The listing builds one solid part. Answer for the finished solid, in the listing's coordinates (mm). Face numbers are marked on the shaded views. A direction names the side the tool comes from. Give positions to 0.01 mm unless a question says otherwise; leave off trailing zeros. Loops run counter-clockwise (first coordinate to the right, second up) from the corner with the lowest first, then second, coordinate; pieces in that order, holes last. Notation, with made-up numbers: (54.25, 66.5) - (105.25, 66.5) arc R24 cw to (105.25, 97.5) - close; hole circle Ø1 at (51, -22). An arc over 180 degrees is marked (long way). One line per item, written item: value. Start each with the question number.
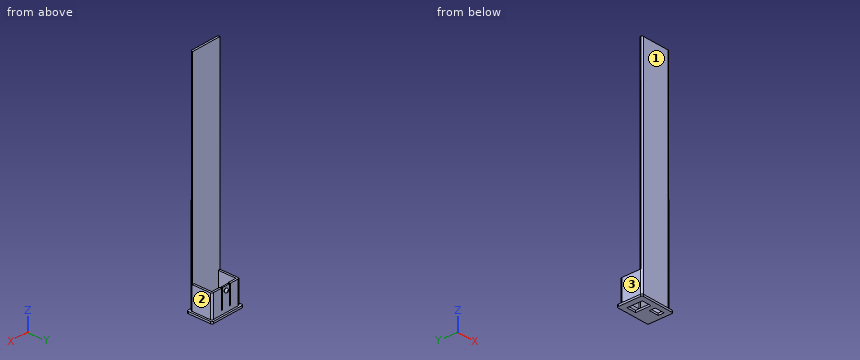
from build123d import *

# Parameters (mm, degrees)
SKETCH1_W           = 25.4
SKETCH1_H           = 17.78
BOSS_EXTRUDE1_DEPTH = 19.05
SKETCH2_W           = 25.4
SKETCH2_H           = 0.79375
BOSS_EXTRUDE2_DEPTH = 165.1
SKETCH3_W           = 28.575
SKETCH3_H           = 20.955
BOSS_EXTRUDE3_DEPTH = 1.5875
SKETCH4_W           = 22.167429019
SKETCH4_H           = 15.39875
CUT_EXTRUDE1_DEPTH  = 19.05
CUT_EXTRUDE2_DEPTH  = 1.5875
SKETCH8_W           = 7.9375
SKETCH8_H           = 4.7625
CUT_EXTRUDE3_DEPTH  = 1.5875
FILLET9_R           = 1.27
FILLET10_R          = 1.27
FILLET11_R          = 1.27
FILLET12_R          = 1.27
FILLET13_R          = 1.27
FILLET14_R          = 1.27
FILLET15_R          = 1.27
FILLET16_R          = 1.27
SKETCH9_W           = 0.79375
SKETCH9_H           = 15.875
CUT_EXTRUDE5_DEPTH  = 1.5875
SKETCH11_W          = 0.79375
SKETCH11_H          = 15.875
CUT_EXTRUDE6_DEPTH  = 1.5875
SKETCH12_W          = 6.50875
SKETCH12_H          = 0.467297544
CUT_EXTRUDE7_DEPTH  = 15.875
SKETCH13_R          = 1.5875
BOSS_EXTRUDE5_DEPTH = 1.5875
FILLET22_R          = 1.27
SKETCH17_W          = 22.167429019
SKETCH17_H          = 19.05
BOSS_EXTRUDE6_DEPTH = 0.79375
SKETCH18_W          = 25.21464302
SKETCH18_H          = 165.1
BOSS_EXTRUDE7_DEPTH = 0.79375


with BuildPart() as part:
    # Sketch1 → Boss-Extrude1 (new body)
    with BuildSketch(Plane.XY):
        with Locations((12.7, 8.89)):
            Rectangle(SKETCH1_W, SKETCH1_H)
    extrude(amount=BOSS_EXTRUDE1_DEPTH)

    # Sketch2 → Boss-Extrude2 (add)
    with BuildSketch(Plane.XY.offset(19.05)):
        with Locations((12.7, 0.396875)):
            Rectangle(SKETCH2_W, SKETCH2_H)
    extrude(amount=BOSS_EXTRUDE2_DEPTH)

    # Sketch3 → Boss-Extrude3 (add)
    with BuildSketch(Plane(origin=(0, 0, 0), x_dir=(-1, 0, 0), z_dir=(0, 0, -1))):
        with Locations((-12.7, 8.89)):
            Rectangle(SKETCH3_W, SKETCH3_H)
    extrude(amount=BOSS_EXTRUDE3_DEPTH)

    # Sketch4 → Cut-Extrude1 (cut)
    with BuildSketch(Plane.XY.offset(19.05)):
        with Locations((12.67121451, 8.493125)):
            Rectangle(SKETCH4_W, SKETCH4_H)
    extrude(amount=-CUT_EXTRUDE1_DEPTH, mode=Mode.SUBTRACT)

    # Sketch5 → Cut-Extrude2 (cut)
    with BuildSketch(Plane(origin=(0, 0, -1.5875), x_dir=(-1, 0, 0), z_dir=(0, 0, -1))):
        Polygon((-11.1125, 15.24), (-11.1125, 8.89), (-11.1125, 2.54), (-3.175, 2.54), (-3.175, 15.24), align=None)
    extrude(amount=-CUT_EXTRUDE2_DEPTH, mode=Mode.SUBTRACT)

    # Sketch8 → Cut-Extrude3 (cut)
    with BuildSketch(Plane(origin=(0, 0, -1.5875), x_dir=(-1, 0, 0), z_dir=(0, 0, -1))):
        with Locations((-19.021212582, 4.92125)):
            Rectangle(SKETCH8_W, SKETCH8_H)
    extrude(amount=-CUT_EXTRUDE3_DEPTH, mode=Mode.SUBTRACT)

    # Fillet9
    fillet9_edges = [part.edges().sort_by_distance(p)[0] for p in [
        (25.4, 17.78, 9.525),
    ]]
    fillet(fillet9_edges, radius=FILLET9_R)

    # Fillet10
    fillet10_edges = [part.edges().sort_by_distance(p)[0] for p in [
        (0, 17.78, 9.525),
    ]]
    fillet(fillet10_edges, radius=FILLET10_R)

    # Fillet11
    # the kernel refuses this fillet: 1.27 mm, written as the material it takes off along each edge
    with BuildSketch(Plane(origin=(25.4, 0, 0), x_dir=(0, 1, 0), z_dir=(0, 0, 1))) as fillet11_piece_1:
        with BuildLine():
            CenterArc((FILLET11_R, FILLET11_R), FILLET11_R, 180, 90)
            Line((0, FILLET11_R), (0, 0))
            Line((0, 0), (FILLET11_R, 0))
        make_face()
    extrude(amount=187.325, mode=Mode.SUBTRACT)

    # Fillet12
    # the kernel refuses this fillet: 1.27 mm, written as the material it takes off along each edge
    with BuildSketch(Plane(origin=(0, 0, 187.325), x_dir=(0, 1, 0), z_dir=(0, 0, -1))) as fillet12_piece_1:
        with BuildLine():
            CenterArc((FILLET12_R, FILLET12_R), FILLET12_R, 180, 90)
            Line((0, FILLET12_R), (0, 0))
            Line((0, 0), (FILLET12_R, 0))
        make_face()
    extrude(amount=187.325, mode=Mode.SUBTRACT)

    # Fillet13
    fillet13_edges = [part.edges().sort_by_distance(p)[0] for p in [
        (-1.5875, -1.5875, -0.79375),
    ]]
    fillet(fillet13_edges, radius=FILLET13_R)

    # Fillet14
    fillet14_edges = [part.edges().sort_by_distance(p)[0] for p in [
        (-1.5875, 19.3675, -0.79375),
    ]]
    fillet(fillet14_edges, radius=FILLET14_R)

    # Fillet15
    fillet15_edges = [part.edges().sort_by_distance(p)[0] for p in [
        (26.9875, -1.5875, -0.79375),
    ]]
    fillet(fillet15_edges, radius=FILLET15_R)

    # Fillet16
    fillet16_edges = [part.edges().sort_by_distance(p)[0] for p in [
        (26.9875, 19.3675, -0.79375),
    ]]
    fillet(fillet16_edges, radius=FILLET16_R)

    # Sketch9 → Cut-Extrude5 (cut)
    with BuildSketch(Plane(origin=(0, 17.78, 0), x_dir=(1, 0, 0), z_dir=(0, 1, 0))):
        with Locations((16.271875, -11.1125)):
            Rectangle(SKETCH9_W, SKETCH9_H)
    extrude(amount=-CUT_EXTRUDE5_DEPTH, mode=Mode.SUBTRACT)

    # Sketch11 → Cut-Extrude6 (cut)
    with BuildSketch(Plane(origin=(0, 17.78, 0), x_dir=(1, 0, 0), z_dir=(0, 1, 0))):
        with Locations((8.969375, -11.1125)):
            Rectangle(SKETCH11_W, SKETCH11_H)
    extrude(amount=-CUT_EXTRUDE6_DEPTH, mode=Mode.SUBTRACT)

    # Sketch12 → Cut-Extrude7 (cut)
    with BuildSketch(Plane.XY.offset(19.05)):
        with Locations((12.620625, 16.426148772)):
            Rectangle(SKETCH12_W, SKETCH12_H)
    extrude(amount=-CUT_EXTRUDE7_DEPTH, mode=Mode.SUBTRACT)

    # Sketch13 → Boss-Extrude5 (add)
    with BuildSketch(Plane(origin=(0, 17.78, 0), x_dir=(1, 0, 0), z_dir=(0, 1, 0))):
        with Locations(Location((12.620625, -15.875, 0), (0, 0, 270))):
            Circle(SKETCH13_R)
    extrude(amount=BOSS_EXTRUDE5_DEPTH)

    # Fillet22
    fillet22_edges = [part.edges().sort_by_distance(p)[0] for p in [
        (12.620625, 19.3675, 14.2875),
    ]]
    fillet(fillet22_edges, radius=FILLET22_R)

    # Sketch17 → Boss-Extrude6 (add)
    with BuildSketch(Plane(origin=(0, 0.79375, 0), x_dir=(1, 0, 0), z_dir=(0, 1, 0))):
        with Locations((12.67121451, -9.525)):
            Rectangle(SKETCH17_W, SKETCH17_H)
    extrude(amount=BOSS_EXTRUDE6_DEPTH)

    # Sketch18 → Boss-Extrude7 (add)
    with BuildSketch(Plane(origin=(0, 0.79375, 0), x_dir=(1, 0, 0), z_dir=(0, 1, 0))):
        with Locations((12.7, -101.6)):
            Rectangle(SKETCH18_W, SKETCH18_H)
    extrude(amount=BOSS_EXTRUDE7_DEPTH)


solid = part.part
1. Flat-ended cylindrical pins translate along their axes: pin 1 (0.6 mm diameter, centred on x = 11.5, y = 17, fed in from +Z); pin 2 (1.2 mm diameter, centred on y = 17, z = 10.5, fed in from -X); pin 3 (5.5 mm diameter, centred on x = 13.5, z = 6, fed in from +Y); pin 4 (2 mm diameter, centred on y = 16.5, z = 21.5, fed in from -X). Find the tip coordinate at first contact, or state that the pin passes through.
2. Find the intervals of material crossed by L1, parallel to X at y = 16.75, z = 9.5 (1 decimal); L2, parallel to Z at x = 2.5, y = 11; L3, parallel to Y at x = 17.25, z = 101.5, in increasing order. Write a range as [from, to].
3. A cutting plane is placed at B-B (z = 162.5). Determine the outline of the cut face in (x, y).
4. For the marked faces 1, 2 and 3, determine the directions among +Z, -Z, +X, -X, +Y, -Y from which every point of the face is accessible in a straight line to the end or side of a thin tool.
Results below:
1. pin 1: stops at z = 19.05
1. pin 2: stops at x = 0
1. pin 3: stops at y = 17.78
1. pin 4: passes through
2. L1: x = [0, 8.6], [9.4, 15.9], [16.7, 25.4]
2. L2: z = [-1.59, 0]
2. L3: y = [0, 1.59]
3. outline: (0.09, 0.79) arc R1.27 ccw to (1.27, 0) - (24.13, 0) arc R1.27 ccw to (25.31, 0.79) - (25.31, 1.59) - (0.09, 1.59) - close
4. face 1: +Z, +X, -X, -Y
4. face 2: +Z, +X, +Y, -Y
4. face 3: +Z, -X, +Y, -Y
